Study the drawing (mm; zero at the part's minimum x, y, z) and answer. A direction names the side the tool comes from. Give positions to 0.01 mm unless a question says otherwise; leave off trailing zeros. Loops run counter-clockwise (first coordinate to the right, second up) from the corner with the lowest first, then second, coordinate; pieces in that order, holes last. Notation, with made-up numbers: (58.5, 26) - (71.5, 26) arc R21 ccw to (71.5, 54) - close; hole circle Ø2 at (76, 27.5). An arc over 180 degrees is marked (long way). One line per item, written item: value. Start each with the question number.
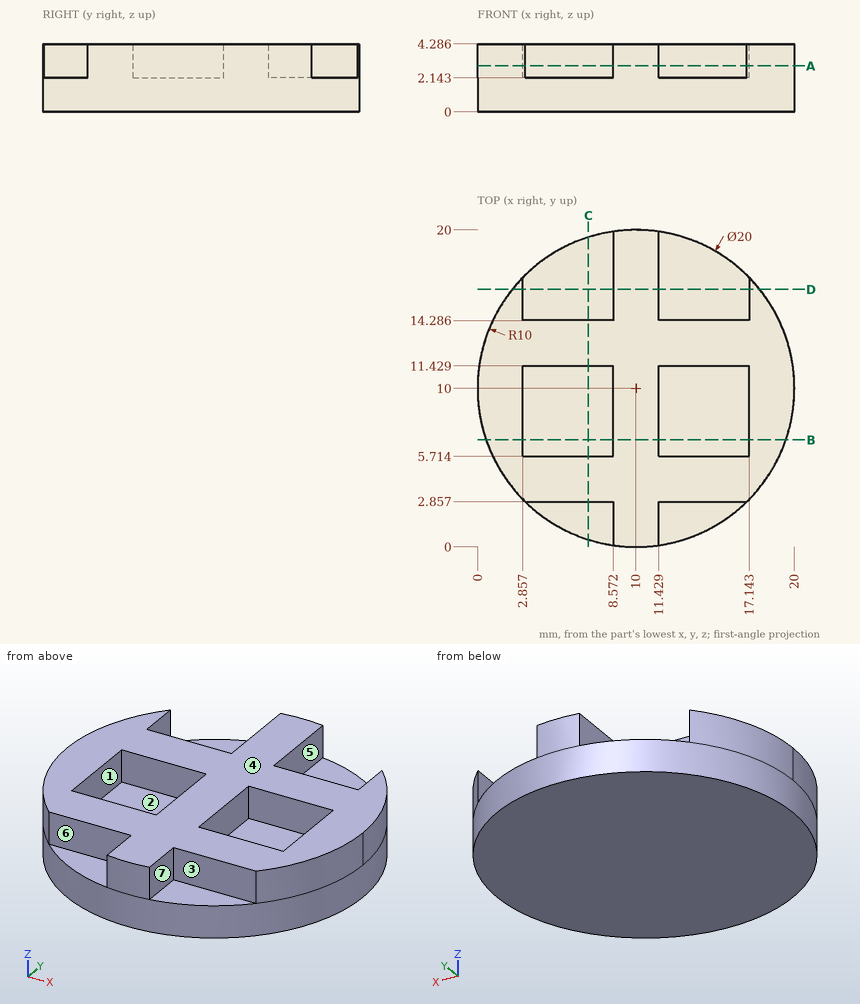
1. A cutting plane is placed at D-D (y = 16.25). Determine the outline of the cut face in (x, z) (1 decimal).
2. A cutting plane is placed at B-B (y = 6.75). Determine the outline of the cut face in (x, z) (1 decimal).
3. A cutting plane is placed at A-A (z = 2.9). Determine the outline of the cut face in (x, y) (1 decimal).
4. Determine the mould class of the marked faces 1, 2, 3 and 4 for opening direction Y: released by +Y, released by -Y, zero draft, split by the parting line, or undercut.
5. Flat-ended cylindrical pins translate along their axes: pin 1 (1.1 mm diameter, centred on x = 13.5, z = 3, fed in from -Y); pin 2 (0.8 mm diameter, centred on x = 15, y = 1.5, fed in from +Z); pin 3 (0.6 mm diameter, centred on x = 5, z = 3.5, fed in from +Y). Find the tip coordinate at first contact, or state that the pin passes through.
6. Find the intervals of material crossed by L1, parallel to Y at x = 15, z = 2.85 (1 decimal); L2, parallel to X at y = 8.75, z = 3.3; L3, parallel to Y at x = 17, z = 1.3, in increasing order. Write a range as [from, to].
7. A cutting plane is placed at C-C (x = 7). Determine the outline of the cut face in (y, z) (1 decimal).
8. For the marked faces 5, 6 and 7, determine the directions among +Z, -Z, +X, -X, +Y, -Y from which every point of the face is accessible in a straight line to the end or side of a thin tool.
Results below:
1. outline: (2.2, 0) - (17.8, 0) - (17.8, 4.3) - (17.1, 4.3) - (17.1, 2.1) - (11.4, 2.1) - (11.4, 4.3) - (8.6, 4.3) - (8.6, 2.1) - (2.9, 2.1) - (2.9, 4.3) - (2.2, 4.3) - close
2. outline: (0.5, 0) - (19.5, 0) - (19.5, 4.3) - (17.1, 4.3) - (17.1, 2.1) - (11.4, 2.1) - (11.4, 4.3) - (8.6, 4.3) - (8.6, 2.1) - (2.9, 2.1) - (2.9, 4.3) - (0.5, 4.3) - close
3. outline: (2.9, 14.3) - (2.9, 17) arc R10 ccw to (3, 2.9) - (8.6, 2.9) - (8.6, 0.1) arc R10 ccw to (11.4, 0.1) - (11.4, 2.9) - (17, 2.9) arc R10 ccw to (17.1, 17) - (17.1, 14.3) - (11.4, 14.3) - (11.4, 19.9) arc R10 ccw to (8.6, 19.9) - (8.6, 14.3) - close; hole (2.9, 5.7) - (8.6, 5.7) - (8.6, 11.4) - (2.9, 11.4) - close; hole (11.4, 5.7) - (17.1, 5.7) - (17.1, 11.4) - (11.4, 11.4) - close
4. face 1: undercut
4. face 2: undercut
4. face 3: released by -Y
4. face 4: zero draft
5. pin 1: stops at y = 2.86
5. pin 2: stops at z = 2.14
5. pin 3: stops at y = 14.29
6. L1: y = [2.9, 5.7], [11.4, 14.3]
6. L2: x = [0.08, 2.86], [8.57, 11.43], [17.14, 19.92]
6. L3: y = [2.86, 17.14]
7. outline: (0.5, 0) - (19.5, 0) - (19.5, 2.1) - (14.3, 2.1) - (14.3, 4.3) - (11.4, 4.3) - (11.4, 2.1) - (5.7, 2.1) - (5.7, 4.3) - (2.9, 4.3) - (2.9, 2.1) - (0.5, 2.1) - close
8. face 5: +Z, +Y
8. face 6: +Z, -X, -Y
8. face 7: +Z, +X, -Y
